Could you check a few things on this model? Use its own coordinates, in mm. Face numbers are marked on the shaded views. Round coordinates to 2 decimals unless told otherwise and drop trailing zeros. Loops run counter-clockwise (first coordinate to the right, second up) from the corner with the lowest first, then second, coordinate; pieces in that order, holes last. Notation, with made-up numbers: (32.5, 32.25) -> (49.5, 32.25) arc R5 cw to (49.5, 40.25) -> close; hole circle Ø7 at (-24, 9.5). An arc over 180 degrees is marked (long way). Write each question's results on one line, items separated by ' | '. Start each with the question number.
1) Imagine slicing it at B-B, the plane y = 0. List the corners of the cut face in (x, z) for me, plus the area to 4 significant figures.
2) We'd pull the mould along Y, two halves only. Please class the marked faces 1, 2 and 3: pulls with the +Y half, pulls with the -Y half, needs draft (parallel to the pull), parting line crosses it, or undercut.
3) Imagine slicing it at A-A, the plane x = 0. List the corners of the cut face in (y, z) for me, plus the area to 3 significant figures.
4) If I drill on probe 1 along Y at (x, z) = (0, 6); probe 2 along Y at (x, z) = (-57, 13.5); probe 3 along Y at (x, z) = (-16, 2.5), over which ranges is the centre line in solid material (lowest first)?
5) Imagine slicing it at D-D, the plane x = -69.5. List the corners of the cut face in (y, z) for me.
6) For P1, Ø8, axis at x = 65, y = 26, coming from the +Z side; P2, Ø3, axis at x = 11, z = 4, coming from the +Y side; P3, Ø5, axis at x = -42, z = 3.5, coming from the -Y side; P4, Ø2, axis at y = -22.5, z = 26, coming from the -X side, each with a flat end and sliding along its axis, tell me the tip position at first contact or that it passes through.
7) Imagine slicing it at C-C, the plane z = 15.5. List the corners of the cut face in (x, y) for me, plus the area to 3 significant figures.
from build123d import *

# Parameters (mm, degrees)
ESBO_O2_R                                      = 86.2
ESBO_O2_R_2                                    = 76.2
RESSALTO_EXTRUS_O1_DEPTH                       = 31
FURO_ROSCADO_PARA_CONDU_TE_DE_M8X1_252_D       = 8.3
FURO_ROSCADO_PARA_CONDU_TE_DE_M8X1_252_DEPTH   = 86.2
FURO_ROSCADO_PARA_CONDU_TE_DE_M8X1_252_O_D     = 8.3
FURO_ROSCADO_PARA_CONDU_TE_DE_M8X1_252_O_DEPTH = 86.2
FURO_ROSCADO_PARA_CONDU_TE_DE_M8X1_2_2_D       = 8.3
FURO_ROSCADO_PARA_CONDU_TE_DE_M8X1_2_2_DEPTH   = 86.2
FURO_ROSCADO_PARA_CONDU_TE_DE_M8X1_2_3_D       = 8.3
FURO_ROSCADO_PARA_CONDU_TE_DE_M8X1_2_3_DEPTH   = 86.2
ESBO_O11_R                                     = 11.25
CORTE_EXTRUS_O1_DEPTH                          = 7.5


with BuildPart() as part:
    # Esboço2 → Ressalto-extrusão1 (new body)
    with BuildSketch(Plane.XY):
        Circle(ESBO_O2_R)
        Circle(ESBO_O2_R_2, mode=Mode.SUBTRACT)
    extrude(amount=RESSALTO_EXTRUS_O1_DEPTH)

    # Furo roscado para conduíte de M8x1.252
    with Locations(Plane(origin=(60.952604538, -60.952604538, 15.5), x_dir=(-0.707106781187, -0.707106781187, 0), z_dir=(0.707106781187, -0.707106781187, 0))):
        with Locations((0, 0)):
            Hole(FURO_ROSCADO_PARA_CONDU_TE_DE_M8X1_252_D / 2, depth=FURO_ROSCADO_PARA_CONDU_TE_DE_M8X1_252_DEPTH)

    # Furo roscado para conduíte de M8x1.252 o
    with Locations(Plane(origin=(-60.952604538, 60.952604538, 15.5), x_dir=(0.707106781187, 0.707106781187, 0), z_dir=(-0.707106781187, 0.707106781187, 0))):
        with Locations((0, 0)):
            Hole(FURO_ROSCADO_PARA_CONDU_TE_DE_M8X1_252_O_D / 2, depth=FURO_ROSCADO_PARA_CONDU_TE_DE_M8X1_252_O_DEPTH)

    # Furo roscado para condu_te de M8x1.2 2
    with Locations(Plane(origin=(60.952604538, 60.952604538, 15.5), x_dir=(0.707106781187, -0.707106781187, 0), z_dir=(0.707106781187, 0.707106781187, 0))):
        with Locations((0, 0)):
            Hole(FURO_ROSCADO_PARA_CONDU_TE_DE_M8X1_2_2_D / 2, depth=FURO_ROSCADO_PARA_CONDU_TE_DE_M8X1_2_2_DEPTH)

    # Furo roscado para condu_te de M8x1.2 3
    with Locations(Plane(origin=(-60.952604538, -60.952604538, 15.5), x_dir=(-0.707106781187, 0.707106781187, 0), z_dir=(-0.707106781187, -0.707106781187, 0))):
        with Locations((0, 0)):
            Hole(FURO_ROSCADO_PARA_CONDU_TE_DE_M8X1_2_3_D / 2, depth=FURO_ROSCADO_PARA_CONDU_TE_DE_M8X1_2_3_DEPTH)

    # Esboço11 → Corte-extrusão1 (cut)
    with BuildSketch(Plane(origin=(86.2, 0, 0), x_dir=(0, 0, -1), z_dir=(1, 0, 0))):
        with Locations((-15.5, 0)):
            Circle(ESBO_O11_R)
    corte_extrus_o1 = extrude(amount=-CORTE_EXTRUS_O1_DEPTH, mode=Mode.SUBTRACT)

    # Espelhar1: Corte-extrusão1 across plane
    add(corte_extrus_o1.mirror(Plane(origin=(0, 0, 0), x_dir=(0, 0, 1), z_dir=(1, 0, 0))), mode=Mode.SUBTRACT)


solid = part.part
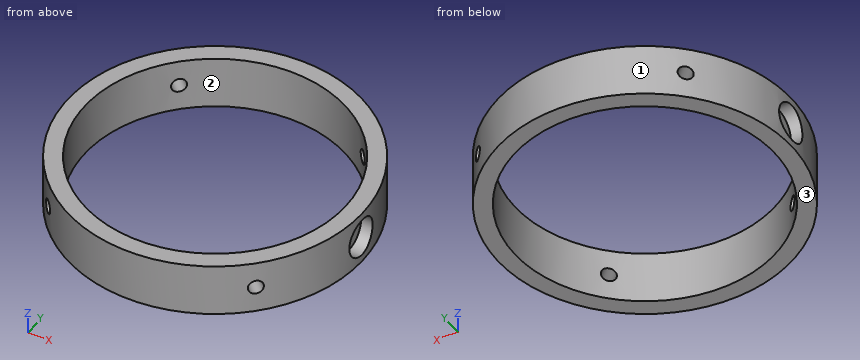
Checked values:
1) outline: (-86.2, 0) -> (-76.2, 0) -> (-76.2, 31) -> (-86.2, 31) -> (-86.2, 26.75) -> (-78.7, 26.75) -> (-78.7, 4.25) -> (-86.2, 4.25) -> close; (76.2, 0) -> (86.2, 0) -> (86.2, 4.25) -> (78.7, 4.25) -> (78.7, 26.75) -> (86.2, 26.75) -> (86.2, 31) -> (76.2, 31) -> close | area: 282.5 mm^2
2) face 1: parting line crosses it | face 2: undercut | face 3: needs draft
3) outline: (-86.2, 0) -> (-76.2, 0) -> (-76.2, 31) -> (-86.2, 31) -> close; (76.2, 0) -> (86.2, 0) -> (86.2, 31) -> (76.2, 31) -> close | area: 620 mm^2
4) probe 1: -86.2 to -76.2, 76.2 to 86.2 | probe 2: -64.66 to -62.14, -51.86 to -50.57, 50.57 to 51.86, 62.14 to 64.66 | probe 3: -84.7 to -74.5, 74.5 to 84.7
5) outline: (-50.99, 0) -> (-31.24, 0) -> (-31.24, 31) -> (-50.99, 31) -> close; (31.24, 0) -> (50.99, 0) -> (50.99, 31) -> (31.24, 31) -> close
6) P1: through | P2: y = 85.67 | P3: y = -76.62 | P4: x = -83.48
7) outline: (-85.46, -11.25) arc R86.2 ccw to (-63.82, -57.95) -> (-56.74, -50.87) arc R76.2 cw to (-56.74, 50.87) -> (-63.82, 57.95) arc R86.2 ccw to (-85.46, 11.25) -> (-78.7, 11.25) -> (-78.7, -11.25) -> close; (-57.95, -63.82) arc R86.2 ccw to (57.95, -63.82) -> (50.87, -56.74) arc R76.2 cw to (-50.87, -56.74) -> close; (-57.95, 63.82) -> (-50.87, 56.74) arc R76.2 cw to (50.87, 56.74) -> (57.95, 63.82) arc R86.2 ccw to start; (56.74, -50.87) -> (63.82, -57.95) arc R86.2 ccw to (85.46, -11.25) -> (78.7, -11.25) -> (78.7, 11.25) -> (85.46, 11.25) arc R86.2 ccw to (63.82, 57.95) -> (56.74, 50.87) arc R76.2 cw to start | area: 4,440 mm^2
